Here's how the part is built. I have some questions about the finished solid (model axes, mm). Face numbers are marked on the shaded views. A direction names the side the tool comes from. Round coordinates to 2 decimals unless told otherwise and drop trailing zeros. Write each loop counter-clockwise with the first axis right and the second up, starting at its lowest first coordinate (ties: lowest second). Pieces come first, ordered by that corner, then holes. Notation, with made-up numbers: M -6.5,1.25 L 32.5,1.25 A13 cw 32.5,12.25 Z; hole C 19,27 d5. An arc over 180 degrees is marked long. Write item = value, one per line. Start each with the question number.
(1) On a 3-axis mill with a long thin cutter (end or side, diameter ignored), from which of +Z, -Z, +X, -X, +Y, -Y can I reach the whole of each face in a straight line? I mean the marked faces 1, 2 and 3. Say none if no direction works.
(2) If we mould it in two halves opening along Z, with no side actions, what happens to the marked faces 4, 5 and 6? For each: released by +Z, released by -Z, zero draft, split by the parting line, or undercut.
(3) I want a section at B-B (z = 4). List the corners of the cut face in (x, y) for me, and give its area (3 significant figures).
(4) I want a section at D-D (x = -10). List the corners of the cut face in (y, z) for me.
(5) Will these pins go through, and if not, where does the flat tip stop? pin 1 Ø10 at (x, y) = (-26, -5) entering from +Z; pin 2 Ø5 at (x, y) = (-4, -1) entering from +Z; pin 3 Ø24.5 at (y, z) = (6.5, 28) entering from -X.
(6) I want a section at C-C (x = 24). List the corners of the cut face in (y, z) for me, and give its area (3 significant figures).
(7) I need wall thicknesses on line 1 along X through (y, z) = (16, 16.5); line 2 along Z through (x, y) = (-12.5, 15.5); line 3 along Z through (x, y) = (-8.5, -13.5). Which ranges of each line are inside material? Lowest first, please.
(8) I want a section at A-A (y = 0). List the corners of the cut face in (x, z) for me.
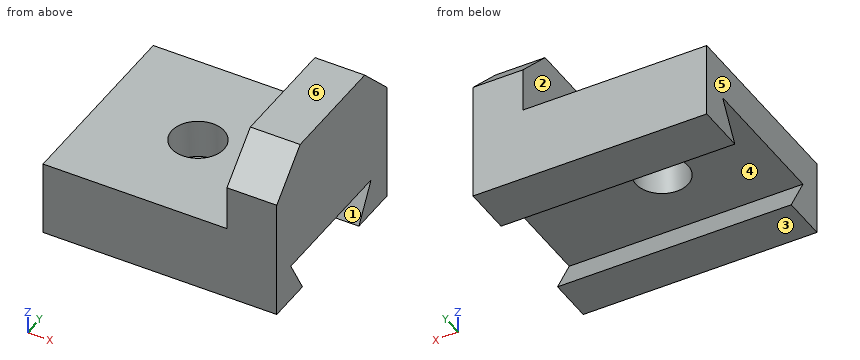
```python
from build123d import *

# Parameters (mm, degrees)
F1_DEPTH      = 25.4
F1_DEPTH_BACK = 25.4
F3_DEPTH      = 25.4
F5_DEPTH      = 108.204
F6_R          = 6.9052604412
F7_DEPTH      = 25.4


with BuildPart() as f1:
    # F0 (on Front) → F1 (new body, two sides)
    with BuildSketch(Plane.XZ) as f1_sk:
        Polygon((16.0311479121, 15.3024597093), (-32.4148759246, 15.3024597093), (-32.4148759246, -4.5178690925), (29.1475392878, -4.5178690925), (29.1475392878, 37.4545902014), (16.0311479121, 37.4545902014), align=None)
    extrude(amount=F1_DEPTH)
    extrude(f1_sk.sketch, amount=-F1_DEPTH_BACK)

    # F2 (on face) → F3 (cut)
    with BuildSketch(Plane(origin=(16.0311479121, 0, 0), x_dir=(0, -1, 0), z_dir=(-1, 0, 0))):
        Polygon((-25.4, 26.9527581858), (-15.1368464701, 37.4545902014), (-25.4, 37.4545902014), align=None)
        Polygon((25.4, 37.4545902014), (14.6135179795, 37.4545902014), (25.4, 27.1370837055), align=None)
    extrude(amount=-F3_DEPTH, mode=Mode.SUBTRACT)

    # F4 (on face) → F5 (cut)
    with BuildSketch(Plane(origin=(-32.4148759246, 0, 0), x_dir=(0, -1, 0), z_dir=(-1, 0, 0))):
        Polygon((13.535389653, -4.5178690925), (18.945902586, 5.1008197479), (-18.0714763701, 5.1008197479), (-12.4605736661, -4.5178690925), align=None)
    extrude(amount=-F5_DEPTH, mode=Mode.SUBTRACT)

    # F6 (on face) → F7 (cut)
    with BuildSketch(Plane.XY.offset(15.3024597093)):
        with Locations((-6.1209849082, 0)):
            Circle(F6_R)
    extrude(amount=-F7_DEPTH, mode=Mode.SUBTRACT)


solid = f1.part
```
Returned:
q1.face_1 = +X, -X
q1.face_2 = +Z, -X, +Y, -Y
q1.face_3 = -Z, +X, -X, +Y, -Y
q2.face_4 = undercut
q2.face_5 = zero draft
q2.face_6 = released by +Z
q3.outline = M -32.41,-25.4 L 29.15,-25.4 L 29.15,-18.33 L -32.41,-18.33 Z; M -32.41,17.43 L 29.15,17.43 L 29.15,25.4 L -32.41,25.4 Z
q3.area = 926 mm²
q4.outline = M -25.4,-4.52 L -13.54,-4.52 L -18.95,5.1 L -5.71,5.1 L -5.71,15.3 L -25.4,15.3 Z; M 5.71,5.1 L 18.07,5.1 L 12.46,-4.52 L 25.4,-4.52 L 25.4,15.3 L 5.71,15.3 Z
q5.pin_1 = 15.3
q5.pin_2 = through
q5.pin_3 = 16.03
q6.outline = M -25.4,-4.52 L -13.54,-4.52 L -18.95,5.1 L 18.07,5.1 L 12.46,-4.52 L 25.4,-4.52 L 25.4,26.95 L 15.14,37.45 L -14.61,37.45 L -25.4,27.14 Z
q6.area = 1,720 mm²
q7.line_1 = 16.03 to 29.15
q7.line_2 = -4.52 to 0.69, 5.1 to 15.3
q7.line_3 = 5.1 to 15.3
q8.outline = M -32.41,5.1 L -13.03,5.1 L -13.03,15.3 L -32.41,15.3 Z; M 0.78,5.1 L 29.15,5.1 L 29.15,37.45 L 16.03,37.45 L 16.03,15.3 L 0.78,15.3 Z
